For this review, take the finished solid that the model builds, in its own axes (mm). Coordinates: 2 decimals unless noted, no trailing zeros. Loops run counter-clockwise (first coordinate to the right, second up) from the corner with the lowest first, then second, coordinate; pieces in that order, holes last. Notation, with made-up numbers: (-28.75, 42) -> (-16.75, 42) arc R26 cw to (-16.75, 61) -> close; hole circle Ø1 at (75, 9.25). An arc over 180 degrees is marked (long way). One line per item, written item: value.
from build123d import *

# Parameters (mm, degrees)
SKETCH1_W               = 1244.6
SKETCH1_H               = 660.4
SKETCH1_W_2             = 666.75
SKETCH1_H_2             = 463.55
BOSS_EXTRUDE1_DEPTH     = 1.2192
F_1_4_CLEARANCE_HOLE1_D = 6.7564


with BuildPart() as part:
    # Sketch1 → Boss-Extrude1 (new body)
    with BuildSketch(Plane(origin=(0, 0, 0), x_dir=(1, 0, 0), z_dir=(0, 1, 0))):
        with Locations((-359.165172795, -51.008449371)):
            Rectangle(SKETCH1_W, SKETCH1_H)
        with Locations((-168.665172795, -51.008449371)):
            Rectangle(SKETCH1_W_2, SKETCH1_H_2, mode=Mode.SUBTRACT)
    extrude(amount=BOSS_EXTRUDE1_DEPTH)

    # 1/4 Clearance Hole1 (through all)
    with Locations(Plane(origin=(0, 0, 0), x_dir=(-1, 0, 0), z_dir=(0, -1, 0))):
        with Locations((968.765172795, 241.091550629), (968.765172795, -51.008449371), (968.765172795, -343.108449371), (644.915172795, -368.508449371), (644.915172795, 266.491550629), (48.015172795, 266.491550629), (-250.434827205, 241.091550629), (-250.434827205, -51.008449371), (-250.434827205, -343.108449371), (48.015172795, -368.508449371)):
            Hole(F_1_4_CLEARANCE_HOLE1_D / 2)


solid = part.part
1. Insertion check: pin 1 Ø5.5 at (x, z) = (250.43, 51.01) entering from -Y. The pin has a flat end and moves straight along its axis. Give the tip position at first contact, or say it passes through.
Return value:
pin 1: passes through
2. Take a section at C-C, the plane y = 0.9. Give the number of separate pieces and of enclosed holes in the cut face, and give its area (3 significant figures).
Return value:
separate pieces: 1
enclosed holes: 11
area: 513,000 mm2
3. Take a section at A-A, the plane z = 18. Give the boundary of the cut face in (x, y).
Return value:
outline: (-981.47, 0) -> (-502.04, 0) -> (-502.04, 1.22) -> (-981.47, 1.22) -> close; (164.71, 0) -> (263.13, 0) -> (263.13, 1.22) -> (164.71, 1.22) -> close
4. Take a section at B-B, the plane x = -449.5. Give the boundary of the cut face in (y, z).
Return value:
outline: (0, -279.19) -> (1.22, -279.19) -> (1.22, -180.77) -> (0, -180.77) -> close; (0, 282.78) -> (1.22, 282.78) -> (1.22, 381.21) -> (0, 381.21) -> close
5. To check wall thickness, follow probe 1 along X at (y, z) = (1.15, 343); probe 2 along X at (y, z) = (1.1, -7.5); probe 3 along Z at (x, y) = (-130.5, 1.05). State the ranges of each line that lie inside material, in increasing order. Write a range as from..to.
Return value:
probe 1: x = -981.47..-972.14, -965.39..247.06, 253.81..263.13
probe 2: x = -981.47..-502.04, 164.71..263.13
probe 3: z = -279.19..-180.77, 282.78..381.21
